from build123d import *

# Parameters (mm, degrees)
SKETCH1_R           = 1.611042105
BOSS_EXTRUDE1_DEPTH = 10
FILLET1_R           = 2


with BuildPart() as part:
    # Sketch1 → Boss-Extrude1 (new body)
    with BuildSketch(Plane(origin=(0, 0, 0), x_dir=(1, 0, 0), z_dir=(0, 1, 0))):
        with BuildLine():
            Line((11.189092539, 48.886576386), (26.189092539, 48.886576386))
            ThreePointArc((26.189092539, 48.886576386), (42.916394787, 44.650618463), (26.189092539, 40.41466054))
            Line((26.189092539, 40.41466054), (11.189092539, 40.41466054))
            Line((11.189092539, 40.41466054), (14.151288092, 30.934521893))
            Line((14.151288092, 30.934521893), (23.265104761, 30.934521893))
            ThreePointArc((23.265104761, 30.934521893), (27.673263401, 29.01898123), (29.280956873, 24.489469079))
            Line((29.280956873, 24.489469079), (38.880945403, 24.489469079))
            ThreePointArc((38.880945403, 24.489469079), (51.981012749, 33.351282464), (67.510407542, 30.354384348))
            ThreePointArc((67.510407542, 30.354384348), (73.416192631, 21.647277215), (79.780316608, 13.269333663))
            ThreePointArc((79.780316608, 13.269333663), (85.455574773, 11.512983879), (89.942117167, 15.407114995))
            ThreePointArc((89.942117167, 15.407114995), (91.312456479, 16.8013043), (93.190330691, 17.344610927))
            Line((93.190330691, 17.344610927), (109.969813161, 17.344610927))
            ThreePointArc((109.969813161, 17.344610927), (114.023930948, 14.937059966), (118.078048735, 17.344610927))
            Line((118.078048735, 17.344610927), (129.094927047, 17.344610927))
            ThreePointArc((129.094927047, 17.344610927), (137.147462695, 24.481469598), (142.365392606, 33.89163907))
            ThreePointArc((142.365392606, 33.89163907), (141.864289866, 37.32830933), (139.079863875, 39.404069031))
            Line((139.079863875, 39.404069031), (121.785643939, 39.404069031))
            Line((121.785643939, 39.404069031), (116.256200304, 36.715011207))
            Line((116.256200304, 36.715011207), (109.969813161, 36.715011207))
            ThreePointArc((109.969813161, 36.715011207), (105.636801382, 39.677321657), (103.958530498, 44.650618463))
            ThreePointArc((103.958530498, 44.650618463), (105.636801382, 49.623915269), (109.969813161, 52.58622572))
            Line((109.969813161, 52.58622572), (116.256200304, 52.58622572))
            Line((116.256200304, 52.58622572), (121.785643939, 49.897167895))
            Line((121.785643939, 49.897167895), (139.079863875, 49.897167895))
            ThreePointArc((139.079863875, 49.897167895), (141.864289866, 51.972927596), (142.365392606, 55.409597857))
            ThreePointArc((142.365392606, 55.409597857), (137.147462695, 64.819767329), (129.094927047, 71.956626))
            Line((129.094927047, 71.956626), (118.078048735, 71.956626))
            ThreePointArc((118.078048735, 71.956626), (114.023930948, 74.364176961), (109.969813161, 71.956626))
            Line((109.969813161, 71.956626), (93.190330691, 71.956626))
            ThreePointArc((93.190330691, 71.956626), (91.312456479, 72.499932627), (89.942117167, 73.894121932))
            ThreePointArc((89.942117167, 73.894121932), (85.455574773, 77.788253047), (79.780316608, 76.031903263))
            ThreePointArc((79.780316608, 76.031903263), (73.416192631, 67.653959712), (67.510407542, 58.946852578))
            ThreePointArc((67.510407542, 58.946852578), (51.981012749, 55.949954462), (38.880945403, 64.811767847))
            Line((38.880945403, 64.811767847), (29.280956873, 64.811767847))
            ThreePointArc((29.280956873, 64.811767847), (27.673263401, 60.282255697), (23.265104761, 58.366715034))
            Line((23.265104761, 58.366715034), (14.151288092, 58.366715034))
            Line((14.151288092, 58.366715034), (11.189092539, 48.886576386))
        make_face()
        with Locations(Location((114.047069209, 69.608036313, 0), (0, 0, 270))):
            Circle(SKETCH1_R, mode=Mode.SUBTRACT)
        with Locations(Location((114.047069209, 19.693200614, 0), (0, 0, 270))):
            Circle(SKETCH1_R, mode=Mode.SUBTRACT)
        with BuildLine():
            Line((100.720147832, 65.775213403), (106.53630451, 65.775213403))
            ThreePointArc((106.53630451, 65.775213403), (108.429983462, 63.84444008), (106.53630451, 61.913666756))
            Line((106.53630451, 61.913666756), (100.720147832, 61.961340172))
            ThreePointArc((100.720147832, 61.961340172), (99.021225351, 63.868276787), (100.720147832, 65.775213403))
        make_face(mode=Mode.SUBTRACT)
        with BuildLine():
            Line((121.585405336, 65.7964452), (127.401562014, 65.7964452))
            ThreePointArc((127.401562014, 65.7964452), (129.295240966, 63.865671877), (127.401562014, 61.934898553))
            Line((127.401562014, 61.934898553), (121.585405336, 61.982571969))
            ThreePointArc((121.585405336, 61.982571969), (119.886482855, 63.889508585), (121.585405336, 65.7964452))
        make_face(mode=Mode.SUBTRACT)
        with BuildLine():
            Line((92.220268628, 53.391525043), (104.709229066, 53.391525043))
            ThreePointArc((104.709229066, 53.391525043), (106.602908018, 55.322298366), (104.709229066, 57.25307169))
            Line((104.709229066, 57.25307169), (92.220268628, 57.205398274))
            ThreePointArc((92.220268628, 57.205398274), (90.521346146, 55.298461659), (92.220268628, 53.391525043))
        make_face(mode=Mode.SUBTRACT)
        with BuildLine():
            Line((122.949689173, 53.478824533), (135.438649611, 53.478824533))
            ThreePointArc((135.438649611, 53.478824533), (137.332328563, 55.409597857), (135.438649611, 57.34037118))
            Line((135.438649611, 57.34037118), (122.949689173, 57.292697765))
            ThreePointArc((122.949689173, 57.292697765), (121.250766691, 55.385761149), (122.949689173, 53.478824533))
        make_face(mode=Mode.SUBTRACT)
        with BuildLine():
            Line((122.949689173, 32.008539162), (135.438649611, 31.960865746))
            ThreePointArc((135.438649611, 31.960865746), (137.332328563, 33.89163907), (135.438649611, 35.822412393))
            Line((135.438649611, 35.822412393), (122.949689173, 35.822412393))
            ThreePointArc((122.949689173, 35.822412393), (121.250766691, 33.915475777), (122.949689173, 32.008539162))
        make_face(mode=Mode.SUBTRACT)
        with BuildLine():
            Line((92.220268628, 32.095838652), (104.709229066, 32.048165237))
            ThreePointArc((104.709229066, 32.048165237), (106.602908018, 33.97893856), (104.709229066, 35.909711883))
            Line((104.709229066, 35.909711883), (92.220268628, 35.909711883))
            ThreePointArc((92.220268628, 35.909711883), (90.521346146, 34.002775268), (92.220268628, 32.095838652))
        make_face(mode=Mode.SUBTRACT)
        with BuildLine():
            Line((121.585405336, 27.318664957), (127.401562014, 27.366338373))
            ThreePointArc((127.401562014, 27.366338373), (129.295240966, 25.43556505), (127.401562014, 23.504791726))
            Line((127.401562014, 23.504791726), (121.585405336, 23.504791726))
            ThreePointArc((121.585405336, 23.504791726), (119.886482855, 25.411728342), (121.585405336, 27.318664957))
        make_face(mode=Mode.SUBTRACT)
        with BuildLine():
            Line((100.720147832, 27.339896755), (106.53630451, 27.38757017))
            ThreePointArc((106.53630451, 27.38757017), (108.429983462, 25.456796847), (106.53630451, 23.526023523))
            Line((106.53630451, 23.526023523), (100.720147832, 23.526023523))
            ThreePointArc((100.720147832, 23.526023523), (99.021225351, 25.432960139), (100.720147832, 27.339896755))
        make_face(mode=Mode.SUBTRACT)
        with BuildLine():
            ThreePointArc((73.357344755, 56.381475255), (77.294040814, 65.186077342), (83.163259717, 72.839237686))
            ThreePointArc((83.163259717, 72.839237686), (86.008327328, 72.620113362), (85.481100389, 69.815749453))
            ThreePointArc((85.481100389, 69.815749453), (80.447104068, 63.142353595), (76.888426245, 55.578548773))
            ThreePointArc((76.888426245, 55.578548773), (74.68795699, 54.067298901), (73.357344755, 56.381475255))
        make_face(mode=Mode.SUBTRACT)
        with BuildLine():
            ThreePointArc((85.481100389, 19.485487474), (80.447104068, 26.158883331), (76.888426245, 33.722688153))
            ThreePointArc((76.888426245, 33.722688153), (74.68795699, 35.233938025), (73.357344755, 32.919761671))
            ThreePointArc((73.357344755, 32.919761671), (77.294040814, 24.115159584), (83.163259717, 16.461999241))
            ThreePointArc((83.163259717, 16.461999241), (86.008327328, 16.681123564), (85.481100389, 19.485487474))
        make_face(mode=Mode.SUBTRACT)
    extrude(amount=BOSS_EXTRUDE1_DEPTH)

    # Fillet1
    fillet1_edges = [part.edges().sort_by_distance(p)[0] for p in [
        (67.510407542, 5, -30.354384348),
        (38.880945403, 5, -24.489469079),
        (29.280956873, 5, -24.489469079),
        (14.151288092, 5, -30.934521893),
        (11.189092539, 5, -40.41466054),
        (11.189092539, 5, -48.886576386),
        (14.151288092, 5, -58.366715034),
        (29.280956873, 5, -64.811767847),
        (38.880945403, 5, -64.811767847),
        (67.510407542, 5, -58.946852578),
        (109.969813161, 5, -71.956626),
        (118.078048735, 5, -71.956626),
        (121.785643939, 5, -49.897167895),
        (116.256200304, 5, -52.58622572),
        (109.969813161, 5, -52.58622572),
        (109.969813161, 5, -36.715011207),
        (116.256200304, 5, -36.715011207),
        (121.785643939, 5, -39.404069031),
        (118.078048735, 5, -17.344610927),
        (109.969813161, 5, -17.344610927),
    ]]
    fillet(fillet1_edges, radius=FILLET1_R)


solid = part.part
Could you check a few things on this model? Use its own coordinates, in mm. A direction names the side the tool comes from. Give positions to 0.01 mm unless a question says otherwise; leave off trailing zeros. Order: outer loops, then holes, each group sorted by start corner. A loop starts at its lowest first (then second) coordinate and runs counter-clockwise, first axis right, second up. Notation, with made-up numbers: M 31.5,-18 L 48.5,-18 A28 cw 48.5,16 Z; hole C -23.5,14.5 d10. An arc over 180 degrees is marked long. One line per question, with ' | ' between items.
1. I want a section at A-A (x = 41). List the corners of the cut face in (y, z) for me.
Results:
outline: M 0,-62.12 L 10,-62.12 L 10,-50.17 L 0,-50.17 Z; M 0,-39.13 L 10,-39.13 L 10,-27.18 L 0,-27.18 Z
2. I'm going to push flat-ended pins straight in: pin 1 (2.5 mm diameter, centred on x = 18.5, y = 2.5, fed in from -Z); pin 2 (1 mm diameter, centred on y = 2, z = -46.5, fed in from -X); pin 3 (6 mm diameter, centred on x = 112.5, y = 5, fed in from +Z). Where does each tip first touch, or does it pass through?
Results:
pin 1: z = -58.37 | pin 2: x = 42.6 | pin 3: z = -14.94
3. We'd pull the mould along X, two halves only. Please class faces 1 (the face through (85.98, 4.93, -72.656)), 2 (the face through (12.87, 4.93, -54.26)), 3 (the face through (19, 5, -30.935)): +X half, -X half, draft (parallel to the pull), parting line (faces both ways), or undercut.
Results:
face 1: undercut | face 2: -X half | face 3: draft
4. I want a section at C-C (y = 7.75). Give the number of separate pieces and of enclosed holes in the cut face, and give its area (3 significant figures).
Results:
separate pieces: 1 | enclosed holes: 12 | area: 4,180 mm²
5. If I drill on line 1 (Z direction, x = 33.5, y = 8.25); line 2 (X direction, y = 2.75, z = -64.5); line 3 (X direction, y = 5.75, z = -29), over which ranges is the centre line in solid material (lowest first)?
Results:
line 1: -64.81 to -53.54, -35.77 to -24.49 | line 2: 30.06 to 38.91, 71.2 to 76.89, 81.3 to 99.13, 108.32 to 119.99, 129.19 to 137.4 | line 3: 27.69 to 42.92, 68.38 to 74.81, 78.88 to 140.18
6. For faces 4 (the face through (119.887, 4.93, -63.85)), 5 (the face through (73.458, 4.93, -21.589)), 6 (the face through (20, 5, -48.887)), which set-ups out of +Z, -Z, +X, -X, +Y, -Y let a thin tool reach every point of the face, with its end or its side?
Results:
face 4: +Y, -Y | face 5: +Z, +Y, -Y | face 6: -X, +Y, -Y
7. I want a section at B-B (x = 96.5). List the corners of the cut face in (y, z) for me, and give its area (3 significant figures).
Results:
outline: M 0,-71.96 L 10,-71.96 L 10,-57.22 L 0,-57.22 Z; M 0,-53.39 L 10,-53.39 L 10,-35.91 L 0,-35.91 Z; M 0,-32.08 L 10,-32.08 L 10,-17.34 L 0,-17.34 Z | area: 470 mm²
8. I want a section at D-D (z = -42.5). List the corners of the cut face in (x, y) for me.
Results:
outline: M 42.65,0 L 104.25,0 L 104.25,10 L 42.65,10 Z
